Design review of the part built by this model. Coordinates are the model's own, in mm. A direction names the side the tool comes from. Coordinates: 2 decimals unless noted, no trailing zeros. Loops run counter-clockwise (first coordinate to the right, second up) from the corner with the lowest first, then second, coordinate; pieces in that order, holes last.
Q1. Add section C-C on x = 69. Give the boundary of the cut face in (y, z).
Q2. For P1, Ø0.9, axis at x = 84.5, z = 2.5, coming from the -Y side, flat-tipped, find the tip position at first contact; note if it passes through.
Q3. Wall thickness on probe 1 along X at (y, z) = (8.5, 2.5); probe 2 along Y at (x, z) = (85, 2.1); probe 3 along Y at (x, z) = (78, 1.55): over which ranges is each line inside the solid? List them lowest first.
Q4. Add section B-B on y = 32. Give the boundary of the cut face in (x, z), and give its area (3 significant figures).
Q5. Add section D-D on y = 11.5. Give the boundary of the cut face in (x, z).
Q6. Machinability: for faces 4 (the face through (4.675, 0.742, 1.036)), 5 (the face through (79.21, 45.897, 2.535)), which of the approach directions +Z, -Z, +X, -X, +Y, -Y give a long, thin tool a straight path to every point of the face, cutting with its end or side? Answer none if there is none.
Q7. Draft analysis for pull direction Z (two halves, no side actions). For faces 1 (the face through (83.5, 11.41, 2.57)), 2 (the face through (44, 22, 0)), 3 (the face through (31.21, 45.897, 2.535)), state which applies: released by +Z, released by -Z, zero draft, split by the parting line, or undercut.
Q8. Add section A-A on x = 5. Give the boundary of the cut face in (y, z).
```python
from build123d import *

# Parameters (mm, degrees)
SKETCH_W        = 90
SKETCH_H        = 55
PAD_DEPTH       = 5
SKETCH001_R     = 9
SKETCH001_R_2   = 12
SKETCH001_R_3   = 2.25
POCKET_DEPTH    = 5
SKETCH002_R     = 1.6
POCKET001_DEPTH = 5
SKETCH003_R     = 1.5
POCKET002_DEPTH = 20


with BuildPart() as part:
    # Sketch → Pad (new body)
    with BuildSketch(Plane.XY):
        with Locations((45, 27.5)):
            Rectangle(SKETCH_W, SKETCH_H)
    extrude(amount=PAD_DEPTH)

    # Sketch001 (on Face6 of Pad) → Pocket (cut)
    with BuildSketch(Plane.XY.offset(5)):
        with Locations((45, 32)):
            Circle(SKETCH001_R)
        with Locations((21, 32)):
            Circle(SKETCH001_R_2)
        with Locations((69, 32)):
            Circle(SKETCH001_R_2)
        with Locations((12, 44)):
            Circle(SKETCH001_R_3)
        with Locations((30, 44)):
            Circle(SKETCH001_R_3)
        with Locations((30, 20)):
            Circle(SKETCH001_R_3)
        with Locations((12, 20)):
            Circle(SKETCH001_R_3)
        with Locations((60, 44)):
            Circle(SKETCH001_R_3)
        with Locations((78, 44)):
            Circle(SKETCH001_R_3)
        with Locations((78, 20)):
            Circle(SKETCH001_R_3)
        with Locations((60, 20)):
            Circle(SKETCH001_R_3)
    extrude(amount=-POCKET_DEPTH, mode=Mode.SUBTRACT)

    # Sketch002 (on Face5 of Pocket) → Pocket001 (cut)
    with BuildSketch(Plane.XY.offset(5)):
        with Locations((5, 52.5)):
            Circle(SKETCH002_R)
        with Locations((5, 2.5)):
            Circle(SKETCH002_R)
        with Locations((85, 2.5)):
            Circle(SKETCH002_R)
        with Locations((85, 52.5)):
            Circle(SKETCH002_R)
        with Locations((5, 42.5)):
            Circle(SKETCH002_R)
        with Locations((85, 42.5)):
            Circle(SKETCH002_R)
    extrude(amount=-POCKET001_DEPTH, mode=Mode.SUBTRACT)

    # Sketch003 (on Face1 of Pocket001) → Pocket002 (cut)
    with BuildSketch(Plane.XZ):
        with Locations((85, 2.5)):
            Circle(SKETCH003_R)
        with Locations((5, 2.5)):
            Circle(SKETCH003_R)
    extrude(amount=-POCKET002_DEPTH, mode=Mode.SUBTRACT)


solid = part.part
```
Entries:
1. outline: (0, 0) - (20, 0) - (20, 5) - (0, 5) - close; (44, 0) - (55, 0) - (55, 5) - (44, 5) - close
2. P1: stops at y = 20
3. probe 1: x = 0 to 3.5, 6.5 to 83.5, 86.5 to 90
3. probe 2: y = 20 to 40.9, 44.1 to 50.9, 54.1 to 55
3. probe 3: y = 0 to 17.75, 22.25 to 24.06, 39.94 to 41.75, 46.25 to 55
4. outline: (0, 0) - (9, 0) - (9, 5) - (0, 5) - close; (33, 0) - (36, 0) - (36, 5) - (33, 5) - close; (54, 0) - (57, 0) - (57, 5) - (54, 5) - close; (81, 0) - (90, 0) - (90, 5) - (81, 5) - close
4. area: 120 mm2
5. outline: (0, 0) - (90, 0) - (90, 5) - (0, 5) - close; hole circle Ø3 at (5, 2.5); hole circle Ø3 at (85, 2.5)
6. face 4: -Y
6. face 5: +Z, -Z
7. face 1: undercut
7. face 2: released by -Z
7. face 3: zero draft
8. outline: (0, 0) - (0.9, 0) - (0.9, 1) - (0, 1) - close; (0, 4) - (0.9, 4) - (0.9, 5) - (0, 5) - close; (4.1, 0) - (40.9, 0) - (40.9, 5) - (4.1, 5) - (4.1, 4) - (20, 4) - (20, 1) - (4.1, 1) - close; (44.1, 0) - (50.9, 0) - (50.9, 5) - (44.1, 5) - close; (54.1, 0) - (55, 0) - (55, 5) - (54.1, 5) - close
